CAD build for the part. Positions are in the model's coordinates, mm. A direction names the side the tool comes from. Round coordinates to 2 decimals unless told otherwise and drop trailing zeros. Loops run counter-clockwise (first coordinate to the right, second up) from the corner with the lowest first, then second, coordinate; pieces in that order, holes last. Notation, with made-up numbers: (-38, 42) -> (-30, 42) arc R23 ccw to (-30, 56) -> close; hole circle Ø7 at (81.5, 72.5). An arc over 180 degrees is marked (long way). Answer as CSV lines item,"result".
```python
from build123d import *

# Parameters (mm, degrees)
CROQUIS1_R              = 2.5
SALIENTE_EXTRUIR1_DEPTH = 5


with BuildPart() as part:
    # Croquis1 → Saliente-Extruir1 (new body)
    # profile 1 of 4: a face of its own
    with BuildSketch(Plane(origin=(0, 0, 0), x_dir=(1, 0, 0), z_dir=(0, 1, 0))):
        Polygon((0, 79), (0, 91), (15, 91), (15, 85), (79, 85), (79, 91), (91, 91), (91, 79), (85, 79), (85, 15), (91, 15), (91, 0), (79, 0), (79, 79), align=None)
        with Locations(Location((85, 85, 0), (0, 0, 270))):
            Circle(CROQUIS1_R, mode=Mode.SUBTRACT)
    # profile 2 of 4: a face of its own
    with BuildSketch(Plane(origin=(0, 0, 0), x_dir=(1, 0, 0), z_dir=(0, 1, 0))):
        Polygon((79, 0), (91, 0), (91, -15), (85, -15), (85, -79), (91, -79), (91, -91), (79, -91), (79, -85), (15, -85), (15, -91), (0, -91), (0, -79), (79, -79), align=None)
        with Locations(Location((85, -85, 0), (0, 0, 270))):
            Circle(CROQUIS1_R, mode=Mode.SUBTRACT)
    # profile 3 of 4: a face of its own
    with BuildSketch(Plane(origin=(0, 0, 0), x_dir=(1, 0, 0), z_dir=(0, 1, 0))):
        Polygon((0, -79), (0, -91), (-15, -91), (-15, -85), (-79, -85), (-79, -91), (-91, -91), (-91, -79), (-85, -79), (-85, -15), (-91, -15), (-91, 0), (-79, 0), (-79, -79), align=None)
        with Locations(Location((-85, -85, 0), (0, 0, 270))):
            Circle(CROQUIS1_R, mode=Mode.SUBTRACT)
    # profile 4 of 4: a face of its own
    with BuildSketch(Plane(origin=(0, 0, 0), x_dir=(1, 0, 0), z_dir=(0, 1, 0))):
        Polygon((0, 79), (-79, 79), (-79, 0), (-91, 0), (-91, 15), (-85, 15), (-85, 79), (-91, 79), (-91, 91), (-79, 91), (-79, 85), (-15, 85), (-15, 91), (0, 91), align=None)
        with Locations(Location((-85, 85, 0), (0, 0, 270))):
            Circle(CROQUIS1_R, mode=Mode.SUBTRACT)
    extrude(amount=SALIENTE_EXTRUIR1_DEPTH)


solid = part.part
```
Q1. Slice it at A-A, the plane z = 43.5. Give the cut face in (x, y).
Results:
outline,"(-85, 0) -> (-79, 0) -> (-79, 5) -> (-85, 5) -> close; (79, 0) -> (85, 0) -> (85, 5) -> (79, 5) -> close"
Q2. Tool access for faces 1 (the flat face through (47, 2, -85)), 2 (the flat face through (88, 2, -79)), 3 (the flat face through (-1, 2, 79)), 4 (the flat face through (-88, 2, 15)): list every direction of +Z, -Z, +X, -X, +Y, -Y with a clear straight run to the whole face (end or side of a thin tool).
Results:
face 1,"-Z, +Y, -Y"
face 2,"+X, +Y, -Y"
face 3,"+Y, -Y"
face 4,"-X, +Y, -Y"
Q3. Probe L1, parallel to X at y = 0.85, z = 9; L2, parallel to Z at x = -49, y = 0.5. List the from-to ranges inside material, lowest first. Write a range as [from, to].
Results:
L1,"[-91, -79], [79, 91]"
L2,"[-85, -79], [79, 85]"
Q4. Drop flat-ended pins along their axis: pin 1 Ø3 at (y, z) = (4, 68.5) entering from -X; pin 2 Ø2.5 at (y, z) = (1.5, -61.5) entering from +X; pin 3 Ø2.5 at (x, y) = (-35, 2.5) entering from -Z. Give the stop position or say it passes through.
Results:
pin 1,"x = -85"
pin 2,"x = 85"
pin 3,"z = -85"
Q5. Two-plate mould, pull along X, no slides. Class faces 5 (the flat face through (-47, 2, 85)), 6 (the flat face through (82, 5, -1)), 7 (the flat face through (-91, 2, 85)): pulls with the +X half, pulls with the -X half, needs draft (parallel to the pull), parting line crosses it, or undercut.
Results:
face 5,"undercut"
face 6,"needs draft"
face 7,"pulls with the -X half"
Q6. Slice it at C-C, the plane y = 4.1. Count the separate pieces of the cut face and the enclosed holes in it, and give its area (3 significant figures).
Results:
separate pieces,"1"
enclosed holes,"5"
area,"5,010 mm2"
Q7. Slice it at B-B, the plane x = -52. Give the cut face in (y, z).
Results:
outline,"(0, -85) -> (5, -85) -> (5, -79) -> (0, -79) -> close; (0, 79) -> (5, 79) -> (5, 85) -> (0, 85) -> close"
